Part model, mm, in its own coordinate system. Coordinates: 2 decimals unless noted, no trailing zeros. Write each loop counter-clockwise with the first axis right and the second up, starting at its lowest first coordinate (ties: lowest second). Pieces come first, ordered by that corner, then holes. Notation, with made-up numbers: M 80,59 L 129,59 A17 ccw 129,84 Z; hole C 34,28 d5. An arc over 180 degrees is marked long. Use a Markdown table: item, result. Add a question column.
Q1. Slice it at D-D on z = 39.5. Write the cut outline in (x, y).
Q2. Pin check, flat tips, straight feed: pin 1 Ø1 at (x, z) = (1.5, -16.5) entering from -Y; pin 2 Ø3 at (y, z) = (-2, -12.5) entering from -X; pin 3 Ø0.6 at (x, z) = (-1.5, -1) entering from +Y. Stop position of each tip, or through.
Q3. Wall check: L1, parallel to X at y = -0.5, z = -16; L2, parallel to Y at x = 1.1, z = 23; L3, parallel to Z at x = 1.1, y = 1.9. Give the ranges that are in metal, low to high. Write a range as from..to.
Q4. Slice it at A-A on y = 0. Write the cut outline in (x, z), then the cut area to 3 significant figures.
Q5. Slice it at B-B on z = 0. Write the cut outline in (x, y).
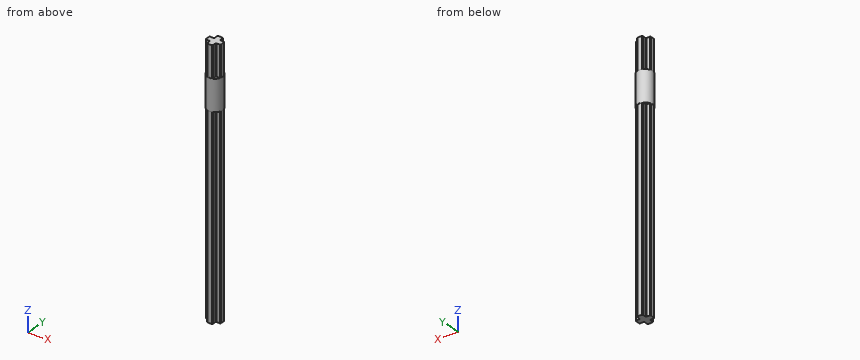
Autodesk Inventor part; units mm, degrees
ref_plane "Plano de trabajo1" through (-15, -5, 43) normal (0, 0, 1) x (1, 0, 0)
ref_plane "Plano de trabajo2" through (-15, -5, 33) normal (0, 0, -1) x (0, 1, 0)
ref_plane "YZ Plane" through (0, 0, 0) normal (1, 0, 0) x (0, 1, 0)
ref_plane "Plano de trabajo3" through (-1.1085, 1.0105, -30.6473) normal (0, 0, 1) x (1, 0, 0)
ref_plane "Plano de trabajo4" through (0, 7, 53) normal (0, 0, 1) x (-1, 0, 0)
sketch "Boceto1" plane through (0, 0, 0) normal (0, 0, 1) x (1, 0, 0)
  line L0 (0.9, -2.4) -> (-0.9, -2.4)
  line L1 (-0.9, -2.4) -> (-0.9, 2.4)
  line L2 (-0.9, 2.4) -> (0.9, 2.4)
  line L3 (0.9, 2.4) -> (0.9, -2.4)
  line L4 (0.9, -2.4) -> (-0.9, 2.4) construction
  line L5 (-0.9, -2.4) -> (0.9, 2.4) construction
  line L6 (2.4, -0.9) -> (-2.4, -0.9)
  line L7 (-2.4, -0.9) -> (-2.4, 0.9)
  line L8 (-2.4, 0.9) -> (2.4, 0.9)
  line L9 (2.4, 0.9) -> (2.4, -0.9)
  line L10 (2.4, -0.9) -> (-2.4, 0.9) construction
  line L11 (-2.4, -0.9) -> (2.4, 0.9) construction
  circle A0 centre (0, 0) radius 1.4
  point P0 (1.0724, 0.9)
  point P1 (0.9, 1.0724)
  point P2 (-0.9, 1.0724)
  point P3 (-1.0724, 0.9)
  point P4 (-1.0724, -0.9)
  point P5 (-0.9, -1.0724)
  point P6 (0.9, -1.0724)
  point P7 (1.0724, -0.9)
  dimension "d0" = 1.8
  dimension "d1" = 4.8
  dimension "d2" = 2.8
extrude "Extrusión1" add sketch "Boceto1" along normal up to surface (83.6473 mm away) from surface at -30.6473
chamfer "Chaflán1" distance 0.2 angle 45 8 edges at (0.9, 2.4, 11.1763) (2.4, 0.9, 11.1763) (2.4, -0.9, 11.1763) (0.9, -2.4, 11.1763) (-0.9, 2.4, 11.1763) (-2.4, 0.9, 11.1763) (-2.4, -0.9, 11.1763) (-0.9, -2.4, 11.1763)
sketch "Boceto2" plane through (0, 0, 53) normal (0, 0, 1) x (1, 0, 0)
  circle A0 centre (0, 0) radius 2.5
  dimension "d8" = 5
ref_plane "Plano de trabajo1" through (-15, -5, 43) normal (0, 0, 1) x (1, 0, 0)
ref_plane "Plano de trabajo2" through (-15, -5, 33) normal (0, 0, -1) x (0, 1, 0)
extrude "Extrusión2" add sketch "Boceto2" against normal up to surface (10 mm away) from surface at -10
properties part number "EjeDelMotor"
Recorded:
| question | item | result |
|---|---|---|
| 1 | outline | C 0,0 d5 |
| 2 | pin 1 | y = -0.98 |
| 2 | pin 2 | x = -2.4 |
| 2 | pin 3 | y = 0.9 |
| 3 | L1 | -2.4..2.4 |
| 3 | L2 | -0.9..0.9 |
| 3 | L3 | 33..43 |
| 4 | outline | M -2.5,33 L -2.4,33 L -2.4,-30.65 L 2.4,-30.65 L 2.4,33 L 2.5,33 L 2.5,43 L 2.4,43 L 2.4,53 L -2.4,53 L -2.4,43 L -2.5,43 Z |
| 4 | area | 404 mm² |
| 5 | outline | M -2.4,-0.7 L -2.2,-0.9 L -1.07,-0.9 A1.4 ccw -0.9,-1.07 L -0.9,-2.2 L -0.7,-2.4 L 0.7,-2.4 L 0.9,-2.2 L 0.9,-1.07 A1.4 ccw 1.07,-0.9 L 2.2,-0.9 L 2.4,-0.7 L 2.4,0.7 L 2.2,0.9 L 1.07,0.9 A1.4 ccw 0.9,1.07 L 0.9,2.2 L 0.7,2.4 L -0.7,2.4 L -0.9,2.2 L -0.9,1.07 A1.4 ccw -1.07,0.9 L -2.2,0.9 L -2.4,0.7 Z |
